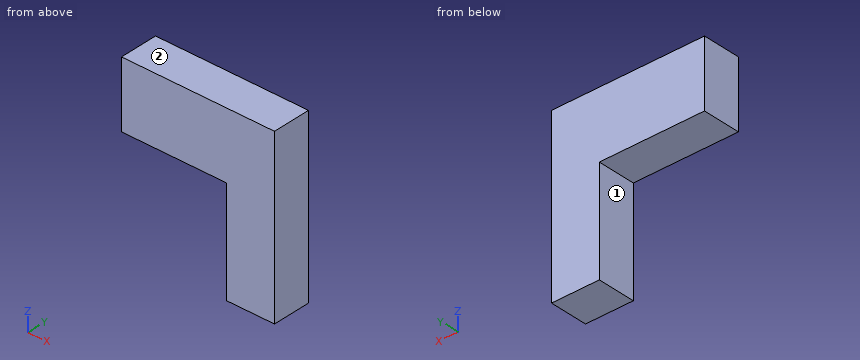
```python
from build123d import *

# Parameters (mm, degrees)
F0_W     = 457.2
F0_H     = 609.6
F1_DEPTH = 101.6
F3_DEPTH = 101.6


with BuildPart() as f1:
    # F0 (on Front) → F1 (new body)
    with BuildSketch(Plane.XZ):
        Rectangle(F0_W, F0_H)
    extrude(amount=F1_DEPTH)

    # F2 (on face) → F3 (cut, through all)
    with BuildSketch(Plane.XZ.offset(101.6)):
        Polygon((101.6, 127), (-177.8, 127), (-177.8, 304.8), (-228.6, 304.8), (-228.6, 127), (-228.6, -304.8), (101.6, -304.8), (228.6, -304.8), (228.6, -152.4), (101.6, -152.4), align=None)
    extrude(amount=-F3_DEPTH, mode=Mode.SUBTRACT)


solid = f1.part
```
Source: CAD feature listing. Evaluate the final solid. Frame: model axes, mm. Face numbers are marked on the shaded views. A direction names the side the tool comes from. Coordinates: 2 decimals unless noted, no trailing zeros. Order: outer loops, then holes, each group sorted by start corner. A loop starts at its lowest first (then second) coordinate and runs counter-clockwise, first axis right, second up. Notation, with made-up numbers: (3.5, -9) - (56.5, -9) arc R11 cw to (56.5, 0) - close; hole circle Ø10 at (31, -39.75). An arc over 180 degrees is marked (long way). One line per item, written item: value.
1) Ray query, line 1 (X direction, y = -26.5, z = 55.5); line 2 (Z direction, x = -32, y = -67). Return the intervals inside material, ascending. Write a range as [from, to].
Computed values:
line 1: x = [101.6, 228.6]
line 2: z = [127, 304.8]
2) Reachability of the marked faces 1 and 2 from +Z, -Z, +X, -X, +Y, -Y: full face, straight path, thin tool, end or side. Return the list, or none.
Computed values:
face 1: -Z, -X, +Y, -Y
face 2: +Z, +X, -X, +Y, -Y
3) Contact query for a flat-ended pin moving along its axis: pin 1 (2 mm diameter, centred on x = -126, y = -79.5, fed in from -Z). Output: stop coordinate, or through.
Computed values:
pin 1: stops at z = 127
4) Cut plane A-A on y = -31.5. Output: boundary loops of the cut face in (x, z), plus the area to 3 significant figures.
Computed values:
outline: (-177.8, 127) - (101.6, 127) - (101.6, -152.4) - (228.6, -152.4) - (228.6, 304.8) - (-177.8, 304.8) - close
area: 108,000 mm^2
5) Cut plane B-B on z = 58. Output: boundary loops of the cut face in (x, y), plus the area to 3 significant figures.
Computed values:
outline: (101.6, -101.6) - (228.6, -101.6) - (228.6, 0) - (101.6, 0) - close
area: 12,900 mm^2
6) Cut plane C-C on x = -10. Output: boundary loops of the cut face in (y, z).
Computed values:
outline: (-101.6, 127) - (0, 127) - (0, 304.8) - (-101.6, 304.8) - close
